Read the model definition and answer for the solid it produces. Units are mm, in the model's axes. Face numbers are marked on the shaded views. Give positions to 0.01 mm unless a question says otherwise; leave off trailing zeros. Write each loop counter-clockwise with the first axis right and the second up, starting at its lowest first coordinate (ties: lowest second). Pieces come first, ordered by that corner, then holes.
Autodesk Inventor part; units mm, degrees
ref_plane "YZ Plane" through (0, 0, 0) normal (1, 0, 0) x (0, 1, 0)
ref_plane "XZ Plane" through (0, 0, 0) normal (0, 1, 0) x (-1, 0, 0)
ref_plane "XY Plane" through (0, 0, 0) normal (0, 0, 1) x (1, 0, 0)
sketch "Schizzo1" plane through (0, 0, 0) normal (1, 0, 0) x (0, 1, 0)
  circle A0 centre (57.5242, -67.0257) radius 11
  line L0 (37.5242, -92.0257) -> (79.5242, -92.0257)
  line L1 (79.5242, -92.0257) -> (79.5242, -42.0257)
  line L2 (79.5242, -42.0257) -> (37.5242, -42.0257)
  line L3 (37.5242, -42.0257) -> (37.5242, -92.0257)
  circle A1 centre (42.0242, -82.5257) radius 1.75
  circle A2 centre (42.0242, -51.5257) radius 1.75
  circle A3 centre (73.0242, -51.5257) radius 1.75
  circle A4 centre (73.0242, -82.5257) radius 1.75
  point P0 (0, 0)
  point P1 (79.5242, -67.0257)
  dimension "d0" = 22
  dimension "d1" = 42
  dimension "d2" = 50
  dimension "d4" = 31
  dimension "d5" = 31
  dimension "d6" = 15.5
  dimension "d7" = 31
  dimension "d8" = 31
  dimension "d9" = 0
  dimension "d10" = 15.5
  dimension "d11" = 0
  dimension "d12" = 3.5
  dimension "d13" = 3.5
  dimension "d14" = 3.5
  dimension "d15" = 3.5
  dimension "d16" = 22
  dimension "d17" = 25
extrude "Estrusione1" add sketch "Schizzo1" along normal blind 10
equation "\"d5\" = d4"
equation "\"d6\" = 0.5 * d4"
equation "\"d7\" = d4"
equation "\"d8\" = d4"
equation "\"d10\" = 0.5 * d4"
equation "\"d13\" = d12"
equation "\"d14\" = d12"
equation "\"d15\" = d12"
equation "\"d17\" = 0.5 * d2"
properties part number "staffa motore"
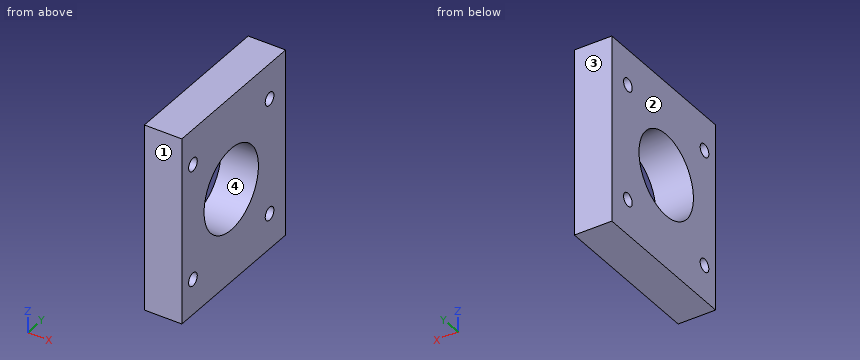
Item 1: Section C-C (x = 6.25) is taken. Write down the section's boundary in (y, z).
Result set:
outline: (37.52, -92.03) - (79.52, -92.03) - (79.52, -42.03) - (37.52, -42.03) - close; hole circle Ø3.5 at (42.02, -82.53); hole circle Ø3.5 at (42.02, -51.53); hole circle Ø22 at (57.52, -67.03); hole circle Ø3.5 at (73.02, -82.53); hole circle Ø3.5 at (73.02, -51.53)
Item 2: Determine the mould class of the marked faces 1, 2, 3 and 4 for opening direction Y: pulls with the +Y half, pulls with the -Y half, needs draft (parallel to the pull), parting line crosses it, or undercut.
Result set:
face 1: pulls with the -Y half
face 2: needs draft
face 3: pulls with the +Y half
face 4: undercut
Item 3: Section A-A (y = 53.5) is taken. Write down the section's boundary in (x, z), and give its area (3 significant figures).
Result set:
outline: (0, -92.03) - (10, -92.03) - (10, -77.26) - (0, -77.26) - close; (0, -56.79) - (10, -56.79) - (10, -42.03) - (0, -42.03) - close
area: 295 mm2
Item 4: Find the intervals of material crossed by line 1 along Z through (x, y) = (8.5, 73); line 2 along Z through (x, y) = (9.5, 71.5); line 3 along Y through (x, z) = (5.75, -83.5), in increasing order.
Result set:
line 1: z = -92.03 to -84.28, -80.78 to -53.28, -49.78 to -42.03
line 2: z = -92.03 to -83.39, -81.67 to -52.39, -50.67 to -42.03
line 3: y = 37.52 to 40.57, 43.48 to 71.57, 74.48 to 79.52
Item 5: This flat-tipped pin is pushed along its axis until it touches: pin 1 Ø5.5 at (y, z) = (73.02, -82.53) entering from +X. Where does it stop, or does it pass through?
Result set:
pin 1: stops at x = 10
Item 6: Section B-B (z = -69) is taken. Write down the section's boundary in (x, y).
Result set:
outline: (0, 37.52) - (10, 37.52) - (10, 46.7) - (0, 46.7) - close; (0, 68.35) - (10, 68.35) - (10, 79.52) - (0, 79.52) - close
